Check sheet for the modelled part. Datum: model origin and axes. Units: mm. A direction names the side the tool comes from. Give positions to 0.01 mm unless a question says otherwise; leave off trailing zeros. Loops run counter-clockwise (first coordinate to the right, second up) from the corner with the lowest first, then second, coordinate; pieces in that order, holes last. Notation, with made-up numbers: M 86,-27.5 L 109,-27.5 A20 ccw 109,2.5 Z; hole C -10.5,86 d4. An arc over 180 degrees is marked long. Use one line per item in the form item = value.
from build123d import *

# Parameters (mm, degrees)
SKETCH1_W                        = 44.45
SKETCH1_H                        = 44.45
SKETCH1_W_2                      = 38.1
SKETCH1_H_2                      = 38.1
BOSS_EXTRUDE1_DEPTH              = 207.16875
BOSS_EXTRUDE1_DEPTH_BACK         = 207.16875
F_17_64_0_26563_DIAMETER_HOLE1_D = 6.747002


with BuildPart() as part:
    # Sketch1 → Boss-Extrude1 (new body, two sides)
    with BuildSketch(Plane(origin=(0, 0, 0), x_dir=(1, 0, 0), z_dir=(0, 1, 0))) as boss_extrude1_sk:
        Rectangle(SKETCH1_W, SKETCH1_H)
        Rectangle(SKETCH1_W_2, SKETCH1_H_2, mode=Mode.SUBTRACT)
    extrude(amount=BOSS_EXTRUDE1_DEPTH)
    extrude(boss_extrude1_sk.sketch, amount=-BOSS_EXTRUDE1_DEPTH_BACK)

    # 17_64 _0.26563_ Diameter Hole1 (through all)
    with Locations(Plane.XY.offset(22.225)):
        with Locations((0, 173.609), (0, -173.609)):
            Hole(F_17_64_0_26563_DIAMETER_HOLE1_D / 2)


solid = part.part
1) Section check C-C (y = 104.5). Record the cut outline in (x, z) (3 decimals).
Evaluation:
outline = M -22.225,-22.225 L 22.225,-22.225 L 22.225,22.225 L -22.225,22.225 Z; hole M -19.05,-19.05 L 19.05,-19.05 L 19.05,19.05 L -19.05,19.05 Z
2) Scan lines: line 1 (Y direction, x = 0, z = -21); line 2 (X direction, y = 94.5, z = 10) (3 decimals). Record each from-to range of solid material in increasing order.
Evaluation:
line_1 = -207.17 to -176.98, -170.24 to 170.24, 176.98 to 207.17
line_2 = -22.225 to -19.05, 19.05 to 22.225
3) Release check for a two-part mould opening along X. For faces 3 (the face through (0.439, -170.264, -20.66)), 4 (the face through (0, 3, 22.225)), 5 (the face through (22.225, 3, 0)) record: pulls with the +X half, pulls with the -X half, needs draft (parallel to the pull), parting line crosses it, or undercut.
Evaluation:
face_3 = undercut
face_4 = needs draft
face_5 = pulls with the +X half
4) Set-up check for faces 1 (the face through (-19.05, 3, 0)), 2 (the face through (0.439, -170.264, 20.615)): record each of +Z, -Z, +X, -X, +Y, -Y from which the full face is reachable in a straight line by a thin tool's end or side.
Evaluation:
face_1 = +Y, -Y
face_2 = +Z, -Z
5) Section check A-A (z = -6.5). Record the cut outline in (x, y) (3 decimals).
Evaluation:
outline = M -22.225,-207.169 L -19.05,-207.169 L -19.05,207.169 L -22.225,207.169 Z; M 19.05,-207.169 L 22.225,-207.169 L 22.225,207.169 L 19.05,207.169 Z
6) Section check B-B (x = 13). Record the cut outline in (y, z) (3 decimals).
Evaluation:
outline = M -207.169,-22.225 L 207.169,-22.225 L 207.169,-19.05 L -207.169,-19.05 Z; M -207.169,19.05 L 207.169,19.05 L 207.169,22.225 L -207.169,22.225 Z
